Verification items for the finished model (mm, model axes). Give positions to 0.01 mm unless a question says otherwise; leave off trailing zeros. Loops run counter-clockwise (first coordinate to the right, second up) from the corner with the lowest first, then second, coordinate; pieces in that order, holes last. Notation, with made-up numbers: (15, 17) - (48, 17) arc R16 ccw to (48, 45) - close; hole circle Ø7 at (20.25, 10). An arc over 180 degrees is marked (long way). One line per question, with ' | ' between items. Start each with the question number.
1. Section check B-B, the plane z = 3.9. State how many separate pieces and enclosed holes the cut face has, then the cut area to 3 significant figures.
2. Depth check by flat-ended pin: pin 1 Ø1 at (x, z) = (-84.5, 1.5) entering from +Y; pin 2 Ø1 at (y, z) = (46, 3.5) entering from -X; pin 3 Ø1.5 at (y, z) = (109.5, 2) entering from -X. Enter the tip coordinate at first touch or a pass-through.
3. Thickness scan on line 1 along Y through (x, z) = (-79, 1.65); line 2 along Y through (x, z) = (0, 1.5); line 3 along X through (y, z) = (-38, 0.6). Record the ranges inside material, lowest first. Write a range as from..to.
4. Section check A-A, the plane y = 78. Enter the section's corners in (x, z), then the cut area to 3 significant figures.
5. Section check C-C, the plane x = -124. Enter the section's corners in (y, z).
6. Section check D-D, the plane y = 19. Enter the section's corners in (x, z).
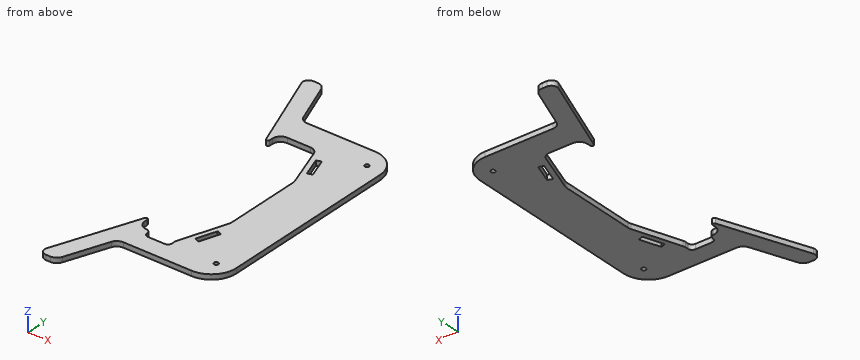
from build123d import *

# Parameters (mm, degrees)
ESBO_O1_R                = 2.6
RESSALTO_EXTRUS_O1_DEPTH = 6
FILETE1_R                = 2
FILETE3_R                = 10
FILETE4_R                = 7
FILETE5_R                = 5
FILETE6_R                = 30


with BuildPart() as part:
    # Esboço1 → Ressalto-extrusão1 (new body)
    with BuildSketch(Plane.XY):
        Polygon((-98.942383725, -137.8), (20, -137.8), (20, 137.8), (-98.942383725, 137.8), (-122.567383725, 200.8), (-145, 200.8), (-100, 80.8), (-100, 105.8), (-55, 105.8), (-35, 47.8), (-35, -47.8), (-55, -105.8), (-55, -115.8), (-85, -115.8), (-85, -105.8), (-100, -105.8), (-100, -80.8), (-145, -200.8), (-122.567383725, -200.8), align=None)
        Polygon((-35.252878569, -66.93878183), (-29.580640679, -68.89472593), (-37.730407762, -92.52905047), (-43.402645652, -90.57310637), align=None, mode=Mode.SUBTRACT)
        Polygon((-43.402645652, 90.57310637), (-37.730407762, 92.52905047), (-29.580640679, 68.89472593), (-35.252878569, 66.93878183), align=None, mode=Mode.SUBTRACT)
        with Locations((0, 113.2)):
            Circle(ESBO_O1_R, mode=Mode.SUBTRACT)
        with Locations((0, -113.2)):
            Circle(ESBO_O1_R, mode=Mode.SUBTRACT)
    extrude(amount=RESSALTO_EXTRUS_O1_DEPTH)

    # Filete1
    filete1_edges = [part.edges().sort_by_distance(p)[0] for p in [
        (-100, -80.8, 3),
        (-100, 80.8, 3),
    ]]
    fillet(filete1_edges, radius=FILETE1_R)

    # Filete3
    filete3_edges = [part.edges().sort_by_distance(p)[0] for p in [
        (-98.942383725, -137.8, 3),
        (-122.567383725, -200.8, 3),
        (-100, -105.8, 3),
        (-55, -105.8, 3),
        (-35, -47.8, 3),
        (-35, 47.8, 3),
        (-55, 105.8, 3),
        (-100, 105.8, 3),
        (-122.567383725, 200.8, 3),
        (-98.942383725, 137.8, 3),
    ]]
    fillet(filete3_edges, radius=FILETE3_R)

    # Filete4
    filete4_edges = [part.edges().sort_by_distance(p)[0] for p in [
        (-145, -200.8, 3),
        (-145, 200.8, 3),
    ]]
    fillet(filete4_edges, radius=FILETE4_R)

    # Filete5
    filete5_edges = [part.edges().sort_by_distance(p)[0] for p in [
        (-85, -115.8, 3),
        (-55, -115.8, 3),
        (-85, -105.8, 3),
    ]]
    fillet(filete5_edges, radius=FILETE5_R - 0.0001)  # a hair under: the kernel refuses the full size

    # Filete6
    filete6_edges = [part.edges().sort_by_distance(p)[0] for p in [
        (20, 137.8, 3),
        (20, -137.8, 3),
    ]]
    fillet(filete6_edges, radius=FILETE6_R)


solid = part.part
Results list:
1) separate pieces: 1 | enclosed holes: 4 | area: 23,500 mm²
2) pin 1: y = 137.8 | pin 2: x = -35.01 | pin 3: x = -111.04
3) line 1: -137.8..-115.8, 105.8..137.8 | line 2: -136.08..-115.8, -110.6..110.6, 115.8..136.08 | line 3: -35..20
4) outline: (-45.41, 0) - (-39.07, 0) - (-39.07, 6) - (-45.41, 6) - close; (-32.72, 0) - (20, 0) - (20, 6) - (-32.72, 6) - close | area: 354 mm²
5) outline: (-199.15, 0) - (-144.8, 0) - (-144.8, 6) - (-199.15, 6) - close; (144.8, 0) - (199.15, 0) - (199.15, 6) - (144.8, 6) - close
6) outline: (-35, 0) - (20, 0) - (20, 6) - (-35, 6) - close
